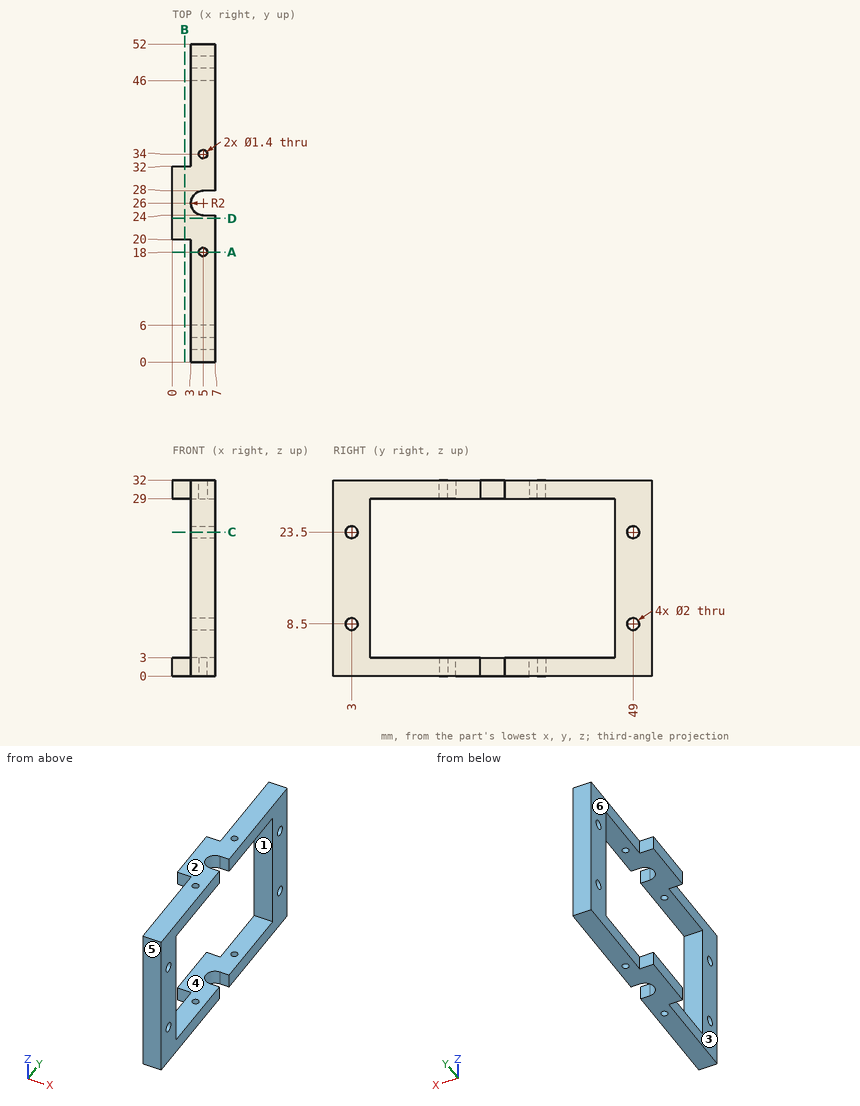
Check sheet for the drawn part. Datum: minimum x, y, z corner. Units: mm. A direction names the side the tool comes from. Round coordinates to 2 decimals unless told otherwise and drop trailing zeros. Order: outer loops, then holes, each group sorted by start corner. A loop starts at its lowest first (then second) coordinate and runs counter-clockwise, first axis right, second up.
1) Section check B-B (x = 2). Record the boundary of the cut face in (y, z).
2) Scan lines: line 1 (Y direction, x = 6.1, z = 8.5); line 2 (Y direction, x = 5, z = 30.55); line 3 (Z direction, x = 5, y = 49). Record each from-to range of solid material in increasing order.
3) Go/stop test with flat-tipped pins: pin 1 Ø3.5 at (x, z) = (1, 31) entering from -Y; pin 2 Ø1.5 at (y, z) = (19, 4) entering from +X; pin 3 Ø2.5 at (y, z) = (49, 23.5) entering from -X. Record where each tip stops, or that it passes through.
4) Mould release check, pull along Z, two halves, no side actions. Record for the marked faces 1, 2 and 3: +Z half, -Z half, draft (parallel to the pull), parting line (faces both ways), or undercut.
5) Section check D-D (y = 23.5). Record the boundary of the cut face in (x, z), and give its area (3 significant figures).
6) Tool access check on the marked faces 4, 5 and 6. Record the directions out of +Z, -Z, +X, -X, +Y, -Y that give a thin tool (end or side, any length) a straight path to the whole face; none if there is none.
7) Section check C-C (z = 23.5). Record the boundary of the cut face in (x, y).
8) Section check A-A (y = 18). Record the boundary of the cut face in (x, z), and give its area (3 significant figures).
Result:
1. outline: (20, 0) - (32, 0) - (32, 3) - (20, 3) - close; (20, 29) - (32, 29) - (32, 32) - (20, 32) - close
2. line 1: y = 0 to 2, 4 to 6, 46 to 48, 50 to 52
2. line 2: y = 0 to 17.3, 18.7 to 24, 28 to 33.3, 34.7 to 52
2. line 3: z = 0 to 7.5, 9.5 to 22.5, 24.5 to 32
3. pin 1: stops at y = 20
3. pin 2: passes through
3. pin 3: stops at x = 3
4. face 1: undercut
4. face 2: +Z half
4. face 3: draft
5. outline: (0, 0) - (7, 0) - (7, 3) - (0, 3) - close; (0, 29) - (7, 29) - (7, 32) - (0, 32) - close
5. area: 42.0 mm2
6. face 4: +X, -X
6. face 5: +Z, -Z, +X, -X, -Y
6. face 6: +Z, -Z, -X, +Y
7. outline: (3, 0) - (7, 0) - (7, 2) - (3, 2) - close; (3, 4) - (7, 4) - (7, 6) - (3, 6) - close; (3, 46) - (7, 46) - (7, 48) - (3, 48) - close; (3, 50) - (7, 50) - (7, 52) - (3, 52) - close
8. outline: (3, 0) - (4.3, 0) - (4.3, 3) - (3, 3) - close; (3, 29) - (4.3, 29) - (4.3, 32) - (3, 32) - close; (5.7, 0) - (7, 0) - (7, 3) - (5.7, 3) - close; (5.7, 29) - (7, 29) - (7, 32) - (5.7, 32) - close
8. area: 15.6 mm2
